from build123d import *

# Parameters (mm, degrees)
F0_R     = 50.8
F1_DEPTH = 25.4
F2_R     = 47.625
F3_DEPTH = 25.4
F4_W     = 38.1
F4_H     = 94.18572
F5_DEPTH = 6.35
F6_W     = 38.1
F6_H     = 46.983762
F7_DEPTH = 6.35


with BuildPart() as f1:
    # F0 (on Front) → F1 (new body)
    with BuildSketch(Plane.XZ):
        Circle(F0_R)
    extrude(amount=-F1_DEPTH)

    # F2 (on face) → F3 (cut)
    with BuildSketch(Plane.XZ):
        Circle(F2_R)
    extrude(amount=-F3_DEPTH, mode=Mode.SUBTRACT)

    # F4 (on face) → F5 (join)
    with BuildSketch(Plane(origin=(0, 25.4, 0), x_dir=(-1, 0, 0), z_dir=(0, 1, 0))):
        Rectangle(F4_W, F4_H)
    extrude(amount=-F5_DEPTH)

    # F6 (on face) → F7 (join)
    with BuildSketch(Plane(origin=(0, 25.4, 0), x_dir=(-1, 0, 0), z_dir=(0, 1, 0))):
        with Locations((0, -52.684718)):
            Rectangle(F6_W, F6_H)
    extrude(amount=F7_DEPTH)


solid = f1.part
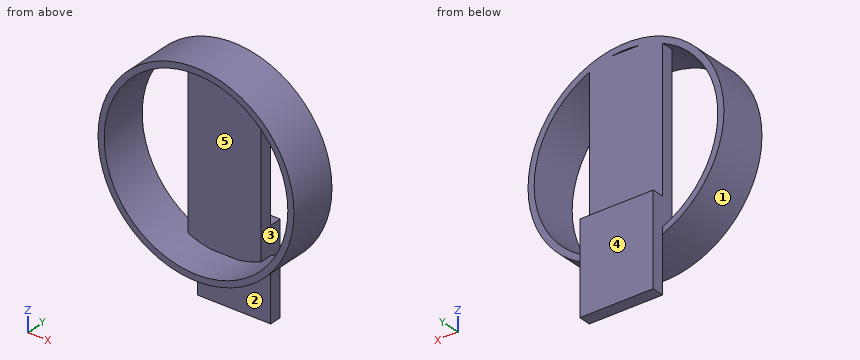
Geometry check sheet. Reference: the model listing, model coordinates, mm. Face numbers are marked on the shaded views. A direction names the side the tool comes from. Round coordinates to 2 decimals unless told otherwise and drop trailing zeros. Loops run counter-clockwise (first coordinate to the right, second up) from the corner with the lowest first, then second, coordinate; pieces in that order, holes last. Notation, with made-up numbers: (83, 9.5) - (90, 9.5) arc R29 cw to (90, 30.5) - close; hole circle Ø11 at (49, -30). An arc over 180 degrees is marked (long way). Answer as CSV lines item,"result".
(1) Cross-section at C-C, the plane y = 27. Enter the section's corners in (x, z), and give its area (3 significant figures).
Output values:
outline,"(-19.05, -76.18) - (19.05, -76.18) - (19.05, -29.19) - (-19.05, -29.19) - close"
area,"1,790 mm²"
(2) Release check for a two-part mould opening along Z. For the marked faces 1, 2 and 3 record: released by +Z, released by -Z, zero draft, split by the parting line, or undercut.
Output values:
face 1,"split by the parting line"
face 2,"zero draft"
face 3,"undercut"
(3) Material ranges on line 1 along X through (y, z) = (10, 0) (3 decimals); line 2 along X through (y, z) = (21.5, 8), recorded low to high.
Output values:
line 1,"x = -50.8 to -47.625, 47.625 to 50.8"
line 2,"x = -50.17 to -46.95, -19.05 to 19.05, 46.95 to 50.17"
(4) Set-up check for the marked faces 4 and 5: record each of +Z, -Z, +X, -X, +Y, -Y from which the full face is reachable in a straight line by a thin tool's end or side.
Output values:
face 4,"+Z, -Z, +X, -X, +Y"
face 5,"-Y"
(5) Depth check by flat-ended pin: pin 1 Ø6 at (y, z) = (21.5, -26) entering from +X; pin 2 Ø3 at (y, z) = (24.5, -49) entering from -X; pin 3 Ø6 at (x, y) = (-12.5, 10) entering from +Z. Enter the tip coordinate at first touch or a pass-through.
Output values:
pin 1,"stops at x = 45.3"
pin 2,"stops at x = -19.05"
pin 3,"stops at z = 49.9"
(6) Cross-section at B-B, the plane z = 0. Enter the section's corners in (x, y) (3 decimals), and give its area (3 significant figures).
Output values:
outline,"(-50.8, 0) - (-47.625, 0) - (-47.625, 25.4) - (-50.8, 25.4) - close; (-19.05, 19.05) - (19.05, 19.05) - (19.05, 25.4) - (-19.05, 25.4) - close; (47.625, 0) - (50.8, 0) - (50.8, 25.4) - (47.625, 25.4) - close"
area,"403 mm²"
(7) Cross-section at D-D, the plane x = 40.5. Enter the section's corners in (y, z).
Output values:
outline,"(0, -30.67) - (25.4, -30.67) - (25.4, -25.06) - (0, -25.06) - close; (0, 25.06) - (25.4, 25.06) - (25.4, 30.67) - (0, 30.67) - close"
(8) Cross-section at A-A, the plane x = 0. Enter the section's corners in (y, z) (3 decimals).
Output values:
outline,"(0, -50.8) - (25.4, -50.8) - (25.4, -76.177) - (31.75, -76.177) - (31.75, -29.193) - (25.4, -29.193) - (25.4, 47.093) - (19.05, 47.093) - (19.05, -47.093) - (25.4, -47.093) - (25.4, -47.625) - (0, -47.625) - close; (0, 47.625) - (25.4, 47.625) - (25.4, 50.8) - (0, 50.8) - close"
